Can you work these out from the model? Positions are in its coordinate system, mm. Face numbers are marked on the shaded views. Round coordinates to 2 decimals unless told otherwise and drop trailing zeros. Order: outer loops, then holes, each group sorted by start corner. A loop starts at its lowest first (then second) coordinate and runs counter-clockwise, first axis right, second up. Notation, with made-up numbers: (-12, 46.25) -> (45, 46.25) arc R28 cw to (45, 74.25) -> close; hole circle Ø1 at (62.5, 1). An arc over 180 degrees is marked (long way). One line per item, written item: value.
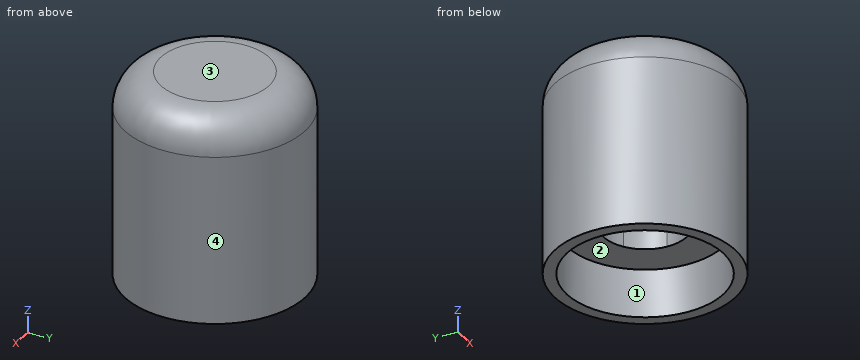
```python
from build123d import *

# Parameters (mm, degrees)
F0_R     = 7.5
F0_R_2   = 6.5
F1_DEPTH = 13
F2_DEPTH = 12
F3_DEPTH = 4
F4_DEPTH = 4
F5_R     = 3


with BuildPart() as f1:
    # F0 (on Top) → F1 (new body)
    with BuildSketch(Plane.XY):
        Circle(F0_R)
        Circle(F0_R_2, mode=Mode.SUBTRACT)
        Circle(F0_R_2)
        with BuildLine():
            ThreePointArc((1.95, 2.8460498942), (3.0520484924, 1.6085707942), (3.45, 0))
            ThreePointArc((3.45, 0), (3.0520484924, -1.6085707942), (1.95, -2.8460498942))
            ThreePointArc((1.95, -2.8460498942), (-3.45, 0), (1.95, 2.8460498942))
        make_face(mode=Mode.SUBTRACT)
        with BuildLine():
            Line((1.95, -2.8460498942), (1.95, 2.8460498942))
            ThreePointArc((1.95, 2.8460498942), (-3.45, 0), (1.95, -2.8460498942))
        make_face()
        with BuildLine():
            ThreePointArc((1.95, -2.8460498942), (3.0520484924, -1.6085707942), (3.45, 0))
            ThreePointArc((3.45, 0), (3.0520484924, 1.6085707942), (1.95, 2.8460498942))
            Line((1.95, 2.8460498942), (1.95, -2.8460498942))
        make_face()
    extrude(amount=F1_DEPTH)

    # F0 (on Top) → F2 (cut)
    with BuildSketch(Plane.XY):
        with BuildLine():
            Line((1.95, -2.8460498942), (1.95, 2.8460498942))
            ThreePointArc((1.95, 2.8460498942), (-3.45, 0), (1.95, -2.8460498942))
        make_face()
    extrude(amount=F2_DEPTH, mode=Mode.SUBTRACT)

    # F0 (on Top) → F3 (cut)
    with BuildSketch(Plane.XY):
        with BuildLine():
            ThreePointArc((1.95, -2.8460498942), (3.0520484924, -1.6085707942), (3.45, 0))
            ThreePointArc((3.45, 0), (3.0520484924, 1.6085707942), (1.95, 2.8460498942))
            Line((1.95, 2.8460498942), (1.95, -2.8460498942))
        make_face()
    extrude(amount=F3_DEPTH, mode=Mode.SUBTRACT)

    # F0 (on Top) → F4 (join)
    with BuildSketch(Plane.XY):
        Circle(F0_R)
        Circle(F0_R_2, mode=Mode.SUBTRACT)
    extrude(amount=-F4_DEPTH)

    # F5
    f5_edges = [f1.edges().sort_by_distance(p)[0] for p in [
        (-7.5, 0, 13),
    ]]
    fillet(f5_edges, radius=F5_R)


solid = f1.part
```
Q1. Will these pins go through, and if not, where does the flat tip stop? pin 1 Ø1 at (x, y) = (-2, -2.5) entering from -Z; pin 2 Ø0.8 at (x, y) = (2.5, -0.5) entering from -Z; pin 3 Ø4 at (x, z) = (4.5, 4) entering from +Y.
Answers below:
pin 1: z = 0
pin 2: z = 4
pin 3: y = 7.07
Q2. I want a section at A-A on z = 9.75. List the corners of the cut face in (x, y) for me.
Answers below:
outline: circle Ø15 at (0, 0); hole (1.95, -2.85) -> (1.95, 2.85) arc R3.45 ccw (long way) to start
Q3. I want a section at C-C on z = -2.5. List the corners of the cut face in (x, y) for me.
Answers below:
outline: circle Ø15 at (0, 0); hole circle Ø13 at (0, 0)
Q4. Please list where these lines run through material, in increasing order: line 1 along Y through (x, z) = (0, -2.2); line 2 along Y through (x, z) = (0, 7.75); line 3 along Z through (x, y) = (2, 3.5).
Answers below:
line 1: -7.5 to -6.5, 6.5 to 7.5
line 2: -7.5 to -3.45, 3.45 to 7.5
line 3: 0 to 13
Q5. We'd pull the mould along X, two halves only. Please class the marked faces 1, 2, 3 and 4: released by +X, released by -X, zero draft, split by the parting line, or undercut.
Answers below:
face 1: undercut
face 2: undercut
face 3: zero draft
face 4: split by the parting line
Q6. I want a section at B-B on x = 0. List the corners of the cut face in (y, z) for me.
Answers below:
outline: (-7.5, -4) -> (-6.5, -4) -> (-6.5, 0) -> (-3.45, 0) -> (-3.45, 12) -> (3.45, 12) -> (3.45, 0) -> (6.5, 0) -> (6.5, -4) -> (7.5, -4) -> (7.5, 10) arc R3 ccw to (4.5, 13) -> (-4.5, 13) arc R3 ccw to (-7.5, 10) -> close
